from build123d import *

# Parameters (mm, degrees)
BOSS_EXTRUDE1_DEPTH = 100
FILLET2_R           = 8
SKETCH2_R           = 30
CUT_EXTRUDE1_DEPTH  = 80


with BuildPart() as part:
    # Sketch1 → Boss-Extrude1 (new body)
    with BuildSketch(Plane(origin=(0, 0, 0), x_dir=(1, 0, 0), z_dir=(0, 1, 0))):
        Polygon((-140, -150), (-140, -350), (140, -350), (140, -150), (215, -150), (215, 150), (-215, 150), (-215, -150), align=None)
    extrude(amount=BOSS_EXTRUDE1_DEPTH)

    # Fillet2
    fillet2_edges = [part.edges().sort_by_distance(p)[0] for p in [
        (140, 50, 350),
        (-140, 50, 350),
        (-215, 50, 150),
        (-215, 50, -150),
        (215, 50, -150),
        (215, 50, 150),
    ]]
    fillet(fillet2_edges, radius=FILLET2_R)

    # Sketch2 → Cut-Extrude1 (cut)
    with BuildSketch(Plane(origin=(0, 100, 0), x_dir=(1, 0, 0), z_dir=(0, 1, 0))):
        Circle(SKETCH2_R)
    extrude(amount=-CUT_EXTRUDE1_DEPTH, mode=Mode.SUBTRACT)


solid = part.part
Work out the finished part from the listing and answer in its coordinate system (mm). A direction names the side the tool comes from. Give positions to 0.01 mm unless a question says otherwise; leave off trailing zeros. Loops run counter-clockwise (first coordinate to the right, second up) from the corner with the lowest first, then second, coordinate; pieces in that order, holes last. Notation, with made-up numbers: M 75,65.5 L 113,65.5 A8 ccw 113,70.5 Z; hole C -16.75,-39 d5. An arc over 180 degrees is marked long. Use CSV: the item, a comma, the result in double quotes.
1) Which of the six approach directions +Z, -Z, +X, -X, +Y, -Y give full straight-line access (tool end or side, diameter ignored) to faces 1 (the flat face through (173, 49, 150)), 2 (the flat face through (-140, 49, 245)), 3 (the flat face through (-215, 49, -2))?
Answer:
face 1,"+Z, +X, +Y, -Y"
face 2,"+Z, -X, +Y, -Y"
face 3,"+Z, -Z, -X, +Y, -Y"
2) Given P1, Ø20, axis at x = -159.5, y = 67, coming from the +Z side; P2, Ø4, axis at x = 54, z = 202, coming from the -Y side, each flat-ended and moving along its own axis, determine where each tip first touches the part or whether it passes through.
Answer:
P1,"z = 150"
P2,"y = 0"
3) Find section C-C on y = 49.5. Write down the section's boundary in (x, z), plus the area to 3 significant figures.
Answer:
outline,"M -215,-142 A8 ccw -207,-150 L 207,-150 A8 ccw 215,-142 L 215,142 A8 ccw 207,150 L 140,150 L 140,342 A8 ccw 132,350 L -132,350 A8 ccw -140,342 L -140,150 L -207,150 A8 ccw -215,142 Z; hole C 0,0 d60"
area,"182,000 mm^2"
4) Consider L1, parallel to X at y = 38, z = 0; L2, parallel to Z at x = 0, y = 57.5; L3, parallel to X at y = 46, z = 304. Determine where each line is inside the solid, lowest interval first.
Answer:
L1,"-215 to -30, 30 to 215"
L2,"-150 to -30, 30 to 350"
L3,"-140 to 140"
5) Find section B-B on z = 0. Write down the section's boundary in (x, y), plus the area to 3 significant figures.
Answer:
outline,"M -215,0 L 215,0 L 215,100 L 30,100 L 30,20 L -30,20 L -30,100 L -215,100 Z"
area,"38,200 mm^2"
6) Find section A-A on y = 14.5. Write down the section's boundary in (x, z), plus the area to 3 significant figures.
Answer:
outline,"M -215,-142 A8 ccw -207,-150 L 207,-150 A8 ccw 215,-142 L 215,142 A8 ccw 207,150 L 140,150 L 140,342 A8 ccw 132,350 L -132,350 A8 ccw -140,342 L -140,150 L -207,150 A8 ccw -215,142 Z"
area,"185,000 mm^2"
7) Determine the mould class of faces 4 (the flat face through (-2, 49, 350)), 5 (the cylindrical face through (-29.97, 60.56, -1.32)), 6 (the flat face through (-3, 0, 41)), 7 (the flat face through (0, 20, 0)) for opening direction Z: released by +Z, released by -Z, zero draft, split by the parting line, or undercut.
Answer:
face 4,"released by +Z"
face 5,"undercut"
face 6,"zero draft"
face 7,"undercut"
8) Find section D-D on x = 0. Write down the section's boundary in (y, z).
Answer:
outline,"M 0,-150 L 100,-150 L 100,-30 L 20,-30 L 20,30 L 100,30 L 100,350 L 0,350 Z"
